```python
from build123d import *

# Parameters (mm, degrees)
SKETCH_1_W          = 10.5
SKETCH_1_H          = 1.3
EXTRUDE_2_DEPTH     = 20
SKETCH_2_R          = 3
SKETCH_2_R_2        = 1.7
EXTRUDE_3_DEPTH     = 5
SKETCH_3_R          = 3
CUT_EXTRUDE_1_DEPTH = 10
SKETCH_4_R          = 1.5
CUT_EXTRUDE_2_DEPTH = 10
FILLET_1_R          = 1


with BuildPart() as part:
    # 草图1 → 凸台-拉伸2 (new body)
    with BuildSketch(Plane(origin=(0, 0, 0), x_dir=(0, 0, -1), z_dir=(1, 0, 0))):
        with Locations((5.25, 0.65)):
            Rectangle(SKETCH_1_W, SKETCH_1_H)
    extrude(amount=EXTRUDE_2_DEPTH)

    # 草图2 → 凸台-拉伸3 (add)
    with BuildSketch(Plane(origin=(20, 0, 0), x_dir=(0, 0, -1), z_dir=(1, 0, 0))):
        with Locations((10.5, 3)):
            Circle(SKETCH_2_R)
        with Locations((10.5, 3)):
            Circle(SKETCH_2_R_2, mode=Mode.SUBTRACT)
    extrude_3 = extrude(amount=-EXTRUDE_3_DEPTH)

    # 草图3 → 切除-拉伸1 (cut)
    with BuildSketch(Plane.ZY.offset(-15)):
        with Locations((-10.5, 3)):
            Circle(SKETCH_3_R)
    extrude(amount=CUT_EXTRUDE_1_DEPTH, mode=Mode.SUBTRACT)

    # 镜向1: 凸台-拉伸3 across plane
    add(extrude_3.mirror(Plane.ZY.offset(-10)))

    # 草图4 → 切除-拉伸2 (cut)
    with BuildSketch(Plane(origin=(0, 1.3, 0), x_dir=(1, 0, 0), z_dir=(0, 1, 0))):
        with Locations((4, 3)):
            Circle(SKETCH_4_R)
    cut_extrude_2 = extrude(amount=-CUT_EXTRUDE_2_DEPTH, mode=Mode.SUBTRACT)

    # 镜向2: 切除-拉伸2 across plane
    add(cut_extrude_2.mirror(Plane.ZY.offset(-10)), mode=Mode.SUBTRACT)

    # 圆角1
    fillet_1_edges = [part.edges().sort_by_distance(p)[0] for p in [
        (20, 0.65, 0),
        (0, 0.65, 0),
    ]]
    fillet(fillet_1_edges, radius=FILLET_1_R)


solid = part.part
```
Verification items for the finished model (mm, model axes). A direction names the side the tool comes from. Coordinates: 2 decimals unless noted, no trailing zeros. Order: outer loops, then holes, each group sorted by start corner. A loop starts at its lowest first (then second) coordinate and runs counter-clockwise, first axis right, second up. Notation, with made-up numbers: (69.5, -37.5) -> (81.5, -37.5) arc R29 ccw to (81.5, 0.5) -> close; hole circle Ø9 at (60, -13.5). An arc over 180 degrees is marked (long way). Put each result on its own line as item: value. Start each with the question number.
1) Cross-section at D-D (y = 5.3). Enter the section's corners in (x, z), plus the area to 3 significant figures.
2) Material ranges on L1, parallel to X at y = 0.8, z = -3; L2, parallel to Z at x = 16.65, y = 3; L3, parallel to X at y = 4.25, z = -8.5, recorded low to high.
3) Cross-section at A-A (x = 4). Enter the section's corners in (y, z), plus the area to 3 significant figures.
4) Cross-section at B-B (z = -3). Enter the section's corners in (x, y), plus the area to 3 significant figures.
5) Tool access check on faces 4 (the flat face through (10, 1, 0)), 5 (the cylindrical face through (10.07, 0.335, -9.122)). Record the directions out of +Z, -Z, +X, -X, +Y, -Y that give a thin tool (end or side, any length) a straight path to the whole face; none if there is none.
6) Release check for a two-part mould opening along X. For faces 1 (the flat face through (10, 1.3, -4)), 2 (the flat face through (20, 2.4, -8.6)), 3 (the flat face through (15, 3, -12.5)) record: pulls with the +X half, pulls with the -X half, needs draft (parallel to the pull), parting line crosses it, or undercut.
7) Cross-section at C-C (y = 3). Enter the section's corners in (x, z).
Geometry check:
1. outline: (0, -12.43) -> (5, -12.43) -> (5, -8.57) -> (0, -8.57) -> close; (15, -12.43) -> (20, -12.43) -> (20, -8.57) -> (15, -8.57) -> close
1. area: 38.5 mm^2
2. L1: x = 0 to 2.5, 5.5 to 14.5, 17.5 to 20
2. L2: z = -13.5 to -12.2, -8.8 to -7.5
2. L3: x = 0 to 5, 15 to 20
3. outline: (0, -10.5) arc R3 ccw (long way) to (1.3, -8.03) -> (1.3, -4.5) -> (0, -4.5) -> close; (0, -1.5) -> (1.3, -1.5) -> (1.3, 0) -> (0, 0) -> close; hole circle Ø3.4 at (3, -10.5)
3. area: 26.7 mm^2
4. outline: (0, 0) -> (2.5, 0) -> (2.5, 1.3) -> (0, 1.3) -> close; (5.5, 0) -> (14.5, 0) -> (14.5, 1.3) -> (5.5, 1.3) -> close; (17.5, 0) -> (20, 0) -> (20, 1.3) -> (17.5, 1.3) -> close
4. area: 18.2 mm^2
5. face 4: +Z, +X, -X, +Y, -Y
5. face 5: -Z, +Y
6. face 1: needs draft
6. face 2: pulls with the +X half
6. face 3: undercut
7. outline: (0, -13.5) -> (5, -13.5) -> (5, -12.2) -> (0, -12.2) -> close; (0, -8.8) -> (5, -8.8) -> (5, -7.5) -> (0, -7.5) -> close; (15, -13.5) -> (20, -13.5) -> (20, -12.2) -> (15, -12.2) -> close; (15, -8.8) -> (20, -8.8) -> (20, -7.5) -> (15, -7.5) -> close
